Geometry: final body of the model. Coordinates: model frame, mm. A direction names the side the tool comes from. Give positions to 0.01 mm unless a question says otherwise; leave off trailing zeros. Loops run counter-clockwise (first coordinate to the right, second up) from the corner with the lowest first, then second, coordinate; pieces in that order, holes last. Notation, with made-up numbers: (29, -37.75) -> (67, -37.75) arc R3 cw to (67, -33.75) -> close; hole circle Ø11 at (-38.5, 30). An arc over 180 degrees is marked (long way). One line per item, written item: value. Start each with the question number.
from build123d import *

# Parameters (mm, degrees)
SKETCH1_R           = 15
BOSS_EXTRUDE1_DEPTH = 20
SKETCH3_R           = 50
BOSS_EXTRUDE2_DEPTH = 20
CHAMFER1_SIZE       = 5
SKETCH4_R           = 4.876598491
SKETCH4_R_2         = 18.007662835
CUT_EXTRUDE1_DEPTH  = 10
SKETCH5_R           = 20
BOSS_EXTRUDE3_DEPTH = 5


with BuildPart() as part:
    # Sketch1 → Boss-Extrude1 (new body)
    with BuildSketch(Plane.XY):
        Circle(SKETCH1_R)
    extrude(amount=BOSS_EXTRUDE1_DEPTH)

    # Sketch3 → Boss-Extrude2 (add)
    with BuildSketch(Plane.XY.offset(20)):
        Circle(SKETCH3_R)
    extrude(amount=BOSS_EXTRUDE2_DEPTH)

    # Chamfer1
    chamfer1_edges = [part.edges().sort_by_distance(p)[0] for p in [
        (-50, 0, 40),
    ]]
    chamfer(chamfer1_edges, length=CHAMFER1_SIZE)

    # Sketch4 → Cut-Extrude1 (cut)
    with BuildSketch(Plane.XY.offset(40)):
        with Locations((27.429667962, 15.836526181)):
            Circle(SKETCH4_R)
        Circle(SKETCH4_R_2)
        with Locations((27.429667962, -15.836526181)):
            Circle(SKETCH4_R)
        with Locations((0, -31.673052363)):
            Circle(SKETCH4_R)
        with Locations((-27.429667961, -15.836526181)):
            Circle(SKETCH4_R)
        with Locations((-27.429667961, 15.836526181)):
            Circle(SKETCH4_R)
        with Locations((0, 31.673052363)):
            Circle(SKETCH4_R)
    extrude(amount=-CUT_EXTRUDE1_DEPTH, mode=Mode.SUBTRACT)

    # Sketch5 → Boss-Extrude3 (add)
    with BuildSketch(Plane(origin=(0, 0, 0), x_dir=(-1, 0, 0), z_dir=(0, 0, -1))):
        Circle(SKETCH5_R)
    extrude(amount=-BOSS_EXTRUDE3_DEPTH)


solid = part.part
Item 1: Section A-A, the plane y = 0. Output: boundary loops of the cut face in (x, z), then the cut area to 3 significant figures.
Item 2: Mould query, pull axis Y, two halves, no side actions, for faces 4 (the face through (-3, 15, 5)), 5 (the face through (0, -32, 30)), 6 (the face through (-14.985, 0.66, 12.395)). Classes: pulls with the +Y half, pulls with the -Y half, needs draft (parallel to the pull), parting line crosses it, or undercut.
Item 3: Pin query (flat end, axial travel): pin 1 (1 mm diameter, centred on y = 12, z = 25, fed in from -X); pin 2 (9 mm diameter, centred on x = -27.43, y = -15.84, fed in from -Z); pin 3 (21.5 mm diameter, centred on x = 0, y = 0, fed in from +Z). Return the tip coordinate at first contact, or that it passes through.
Item 4: Access query for faces 1 (the face through (4.336, -19.524, 2.465)), 2 (the face through (-0.63, 36.51, 35.07)), 3 (the face through (47.69, 15.02, 27.4)). Directions: +Z, -Z, +X, -X, +Y, -Y. A direction counts if a zero-diameter tool reaches every point of the face in a straight line with its end or side. Return the directions, or none.
Item 5: Section B-B, the plane x = 0. Output: boundary loops of the cut face in (y, z).
Item 6: Section C-C, the plane z = 26. Output: boundary loops of the cut face in (x, y).
Item 7: Ray query, line 1 along Y through (x, z) = (0, 33); line 2 along Z through (x, y) = (-25.5, -13.5); line 3 along X through (y, z) = (-2.5, 33). Return the intervals inside material, ascending. Write a range as [from, to].
Item 8: Section D-D, the plane z = 13. Output: boundary loops of the cut face in (x, y), then the cut area to 3 significant figures.
Geometry check:
1. outline: (-50, 20) -> (-15, 20) -> (-15, 5) -> (-20, 5) -> (-20, 0) -> (20, 0) -> (20, 5) -> (15, 5) -> (15, 20) -> (50, 20) -> (50, 35) -> (45, 40) -> (18.01, 40) -> (18.01, 30) -> (-18.01, 30) -> (-18.01, 40) -> (-45, 40) -> (-50, 35) -> close
1. area: 2,260 mm2
2. face 4: needs draft
2. face 5: undercut
2. face 6: parting line crosses it
3. pin 1: stops at x = -48.66
3. pin 2: stops at z = 20
3. pin 3: stops at z = 30
4. face 1: -Z
4. face 2: +Z
4. face 3: +Z, -Z
5. outline: (-50, 20) -> (-15, 20) -> (-15, 5) -> (-20, 5) -> (-20, 0) -> (20, 0) -> (20, 5) -> (15, 5) -> (15, 20) -> (50, 20) -> (50, 35) -> (45, 40) -> (36.55, 40) -> (36.55, 30) -> (26.8, 30) -> (26.8, 40) -> (18.01, 40) -> (18.01, 30) -> (-18.01, 30) -> (-18.01, 40) -> (-26.8, 40) -> (-26.8, 30) -> (-36.55, 30) -> (-36.55, 40) -> (-45, 40) -> (-50, 35) -> close
6. outline: circle Ø100 at (0, 0)
7. line 1: y = [-50, -36.55], [-26.8, -18.01], [18.01, 26.8], [36.55, 50]
7. line 2: z = [20, 30]
7. line 3: x = [-49.94, -17.83], [17.83, 49.94]
8. outline: circle Ø30 at (0, 0)
8. area: 707 mm2
